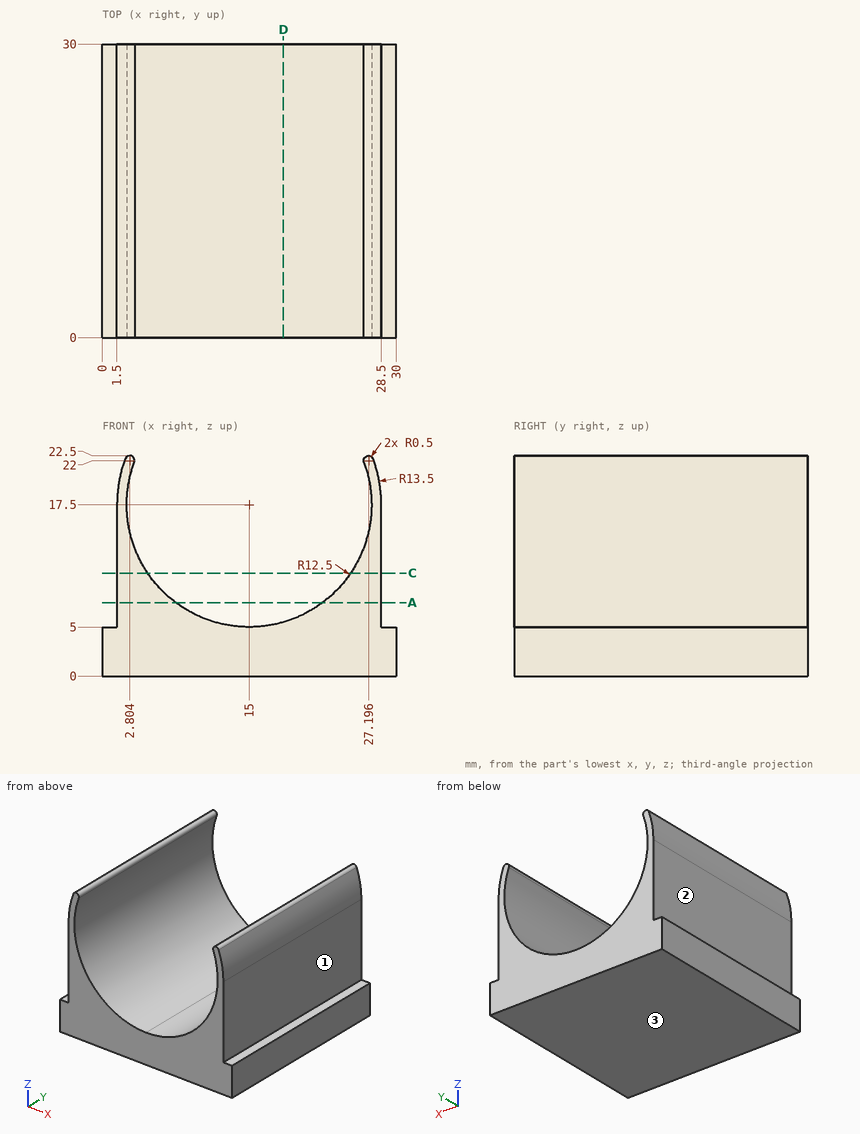
Study the drawing (mm; zero at the part's minimum x, y, z) and answer. A direction names the side the tool comes from. Give positions to 0.01 mm unless a question says otherwise; leave off trailing zeros. Order: outer loops, then holes, each group sorted by start corner. A loop starts at its lowest first (then second) coordinate and runs counter-clockwise, first axis right, second up. Notation, with made-up numbers: M -1.75,18 L 33.25,18 A23 cw 33.25,51 Z; hole C 11,63 d7. An arc over 180 degrees is marked long. Put each result on its own line as item: value. Start each with the question number.
Item 1: Which of the six approach directions +Z, -Z, +X, -X, +Y, -Y give full straight-line access (tool end or side, diameter ignored) to the marked faces 1, 2 and 3?
Item 2: The part is cut by section D-D, the plane x = 18.5. Determine the outline of the cut face in (y, z).
Item 3: The part is cut by section C-C, the plane z = 10.5. Determine the outline of the cut face in (x, y), and give its area (3 significant figures).
Item 4: Flat-ended cylindrical pins translate along their axes: P1, Ø4, axis at y = 18.5, z = 11, coming from the -X side; P2, Ø4, axis at y = 11.5, z = 9.5, coming from the +X side; P3, Ø0.8, axis at x = 29.5, y = 16.5, coming from the +Z side. Find the tip coordinate at first contact, or state that the pin passes through.
Item 5: The part is cut by section A-A, the plane z = 7.5. Determine the outline of the cut face in (x, y), and give its area (3 significant figures).
Item 6: Find the intervals of material crossed by line 1 along X through (y, z) = (17.5, 8.25); line 2 along X through (y, z) = (5, 8) (1 decimal); line 3 along Z through (x, y) = (28.75, 20), in increasing order.
Answer key:
1. face 1: +Z, +X, +Y, -Y
1. face 2: +Z, -X, +Y, -Y
1. face 3: -Z, +X, -X, +Y, -Y
2. outline: M 0,0 L 30,0 L 30,5.5 L 0,5.5 Z
3. outline: M 1.5,0 L 4.64,0 L 4.64,30 L 1.5,30 Z; M 25.36,0 L 28.5,0 L 28.5,30 L 25.36,30 Z
3. area: 189 mm²
4. P1: stops at x = 1.5
4. P2: stops at x = 28.5
4. P3: stops at z = 5
5. outline: M 1.5,0 L 7.5,0 L 7.5,30 L 1.5,30 Z; M 22.5,0 L 28.5,0 L 28.5,30 L 22.5,30 Z
5. area: 360 mm²
6. line 1: x = 1.5 to 6.59, 23.41 to 28.5
6. line 2: x = 1.5 to 6.9, 23.1 to 28.5
6. line 3: z = 0 to 5
